from build123d import *

# Parameters (mm, degrees)
F1_DEPTH  = 76.2
F2_W      = 19.05
F2_H      = 76.2
F3_DEPTH  = 25.4
F3_FACE_W = 19.05
F3_FACE_H = 76.2
F4_DEPTH  = 38.1
F5_R      = 16.51
F6_DEPTH  = 44.45


with BuildPart() as f1:
    # F0 (on Right) → F1 (new body)
    with BuildSketch(Plane.YZ):
        with BuildLine():
            Line((22.535029, 15.43837), (-27.689042, 15.43837))
            ThreePointArc((-27.689042, 15.43837), (-72.957545, -3.900003), (-23.955365, -8.59003))
            Line((-23.955365, -8.59003), (18.801352, -8.59003))
            ThreePointArc((18.801352, -8.59003), (67.803532, -3.900003), (22.535029, 15.43837))
        make_face()
    extrude(amount=F1_DEPTH)

    # F2 (on face) → F3 (join)
    with BuildSketch(Plane(origin=(0, 0, -8.59003), x_dir=(1, 0, 0), z_dir=(0, 0, -1))):
        with Locations((40.256006, 0)):
            Rectangle(F2_W, F2_H)
    extrude(amount=F3_DEPTH)

    # F3_face (on face) → F4 (cut)
    with BuildSketch(Plane(origin=(40.256006, 0, -33.99003), x_dir=(1, 0, 0), z_dir=(0, 0, -1))):
        Rectangle(F3_FACE_W, F3_FACE_H)
    extrude(amount=-F4_DEPTH, mode=Mode.SUBTRACT)

    # F5 (on face) → F6 (cut)
    with BuildSketch(Plane(origin=(0, 0, 0), x_dir=(0, -1, 0), z_dir=(-1, 0, 0))):
        with Locations((-42.704728, 0)):
            Circle(F5_R)
        with Locations((47.858741, 0)):
            Circle(F5_R)
    extrude(amount=-F6_DEPTH, mode=Mode.SUBTRACT)


solid = f1.part
Input: part model. Units: mm. Frame: model coordinates. A direction names the side the tool comes from. Round coordinates to 2 decimals unless told otherwise and drop trailing zeros. Write each loop counter-clockwise with the first axis right and the second up, starting at its lowest first coordinate (ties: lowest second). Pieces come first, ordered by that corner, then holes.
1) Contact query for flat-ended pins moving along their axis: P1, Ø5, axis at x = 33, z = 7.5, coming from the -Y side; P2, Ø9.5, axis at x = 40, y = 14.5, coming from the -Z side; P3, Ø10, axis at x = 47, z = -10, coming from the +Y side. Output: stop coordinate, or through.
2) Cut plane C-C (x = 9.5). Return the cut outline in (y, z), then the cut area to 3 significant figures.
3) Reachability of faces 1 (the flat face through (44.45, -52, 0)), 2 (the flat face through (42, 38.1, -17)), 3 (the flat face through (38, -2, 15.438)), 4 (the flat face through (0, -4, 0)), 5 (the flat face through (15, -3, -8.59)) from +Z, -Z, +X, -X, +Y, -Y: full face, straight path, thin tool, end or side. Return the list, or none.
4) Cut plane D-D (y = -34). Return the cut outline in (x, z).
5) Ray query, L1, parallel to Y at x = 11, z = 0; L2, parallel to Z at x = 42, y = -48.5. Return the intervals inside material, ascending.
6) Cut plane A-A (z = 0). Return the cut outline in (x, y).
7) Draft query along Y for faces 6 (the cylindrical face through (21.914, -63.606, 4.959)), 7 (the flat face through (40, -1, 4.11)), 8 (the flat face through (76.2, -4, 0)). Return one class per face: pulls with the +Y half, pulls with the -Y half, needs draft (parallel to the pull), parting line crosses it, or undercut.
8) Cut plane B-B (y = 13). Return the cut outline in (x, z).
Geometry says:
1. P1: stops at y = -72.76
1. P2: stops at z = 4.11
1. P3: stops at y = 67.61
2. outline: (-27.69, 15.44) arc R25.4 ccw (long way) to (-23.96, -8.59) - (18.8, -8.59) arc R25.4 ccw (long way) to (22.54, 15.44) - close; hole circle Ø33.02 at (-47.86, 0); hole circle Ø33.02 at (42.7, 0)
2. area: 3,360 mm2
3. face 1: -X
3. face 2: -Z
3. face 3: +Z, +X, -X
3. face 4: +Z, -Z, -X, +Y, -Y
3. face 5: -Z, +X, -X
4. outline: (0, -21.29) - (30.73, -21.29) - (30.73, -8.97) - (0, -8.97) - close; (0, 8.97) - (44.45, 8.97) - (44.45, 4.11) - (49.78, 4.11) - (49.78, -21.29) - (76.2, -21.29) - (76.2, 21.29) - (0, 21.29) - close
5. L1: y = -73.26 to -64.37, -31.35 to 26.19, 59.21 to 68.1
5. L2: z = -25.39 to -16.5, 16.5 to 25.39
6. outline: (0, -73.26) - (76.2, -73.26) - (76.2, 68.1) - (0, 68.1) - (0, 59.21) - (44.45, 59.21) - (44.45, 38.1) - (49.78, 38.1) - (49.78, -38.1) - (44.45, -38.1) - (44.45, -64.37) - (0, -64.37) - close; (0, -31.35) - (30.73, -31.35) - (30.73, 26.19) - (0, 26.19) - close
7. face 6: undercut
7. face 7: undercut
7. face 8: needs draft
8. outline: (0, -8.59) - (30.73, -8.59) - (30.73, 4.11) - (49.78, 4.11) - (49.78, -8.59) - (76.2, -8.59) - (76.2, 15.44) - (0, 15.44) - close
